```python
from build123d import *

# Parameters (mm, degrees)
F1_DEPTH = 3.5
F2_R     = 0.15
F4_DEPTH = 25


with BuildPart() as f1:
    # F0 (on Top) → F1 (new body)
    with BuildSketch(Plane.XY):
        with BuildLine():
            ThreePointArc((2.0309193372, 2.850502876), (0, 4.9428488608), (-2.0309193372, 2.850502876))
            ThreePointArc((-2.0309193372, 2.850502876), (0, -3.5), (2.0309193372, 2.850502876))
        make_face()
        with BuildLine():
            ThreePointArc((0.7830913136, 1.8403173625), (0, -2), (-0.7830913136, 1.8403173625))
            ThreePointArc((-0.7830913136, 1.8403173625), (0, 3.4622241035), (0.7830913136, 1.8403173625))
        make_face(mode=Mode.SUBTRACT)
    extrude(amount=F1_DEPTH)

    # F2
    f2_edges = [f1.edges().sort_by_distance(p)[0] for p in [
        (-0.783091, 1.840317, 1.75),
        (0.783091, 1.840317, 1.75),
    ]]
    fillet(f2_edges, radius=F2_R)

    # F3 (on Front) → F4 (cut)
    with BuildSketch(Plane.XZ):
        Polygon((-2.6012919649, 8.286720852), (-4.2398504038, 8.1655834162), (3.1280116344, -5.5110100095), (4.8318293002, -5.5110100095), align=None)
    extrude(amount=F4_DEPTH, mode=Mode.SUBTRACT)


solid = f1.part
```
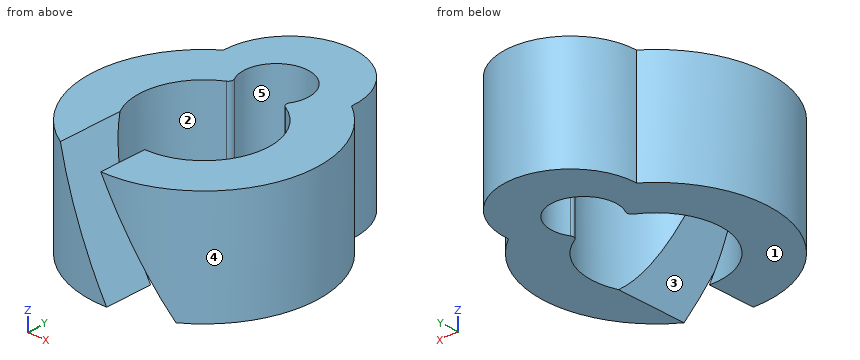
Input: part model. Units: mm. Frame: model coordinates. Face numbers are marked on the shaded views. A direction names the side the tool comes from. Give positions to 0.01 mm unless a question says otherwise; leave off trailing zeros. Write each loop counter-clockwise with the first axis right and the second up, starting at its lowest first coordinate (ties: lowest second). Pieces come first, ordered by that corner, then holes. Notation, with made-up numbers: (33.5, 17) - (57.5, 17) arc R15 ccw to (57.5, 26) - close; hole circle Ø1 at (72, -28). An arc over 180 degrees is marked (long way). Write item = value, one per line. Start each with the question number.
1. Ray query, L1, parallel to X at y = 0, z = 3; L2, parallel to Y at x = 0, z = 2.45; L3, parallel to X at y = -0.5, z = 1.85. Return the intervals inside material, ascending.
2. First-contact query: pin 1 Ø2 at (x, z) = (-1.5, 2) entering from +Y; pin 2 Ø2 at (y, z) = (3, 2.5) entering from +X. Flat tips, straight axial feed; report the tip coordinate or a pass-through.
3. Access query for the marked faces 1 and 2. Directions: +Z, -Z, +X, -X, +Y, -Y. A direction counts if a zero-diameter tool reaches every point of the face in a straight line with its end or side. Return the directions, or none.
4. Section query A-A, the plane y = 2.75. Output: boundary loops of the cut face in (x, z), then the cut area to 3 significant figures.
5. Section query C-C, the plane x = -3. Output: boundary loops of the cut face in (y, z).
6. Section query D-D, the plane x = 2.5. Output: boundary loops of the cut face in (y, z), then the cut area to 3 significant figures.
7. Section query B-B, the plane x = 1.75. Output: boundary loops of the cut face in (y, z).
8. Mould query, pull axis Y, two halves, no side actions, for the marked faces 3, 4 and 5. Classes: released by +Y, released by -Y, zero draft, split by the parting line, or undercut.
Check sheet entries:
q1.L1 = -3.5 to -2, 2 to 3.5
q1.L2 = 3.46 to 4.94
q1.L3 = -3.46 to -1.94, 1.94 to 3.46
q2.pin_1 = 4.88
q2.pin_2 = 2.87
q3.face_1 = -Z, +X, -X, +Y, -Y
q3.face_2 = +Z, -Z
q4.outline = (-2.17, 0) - (-0.96, 0) - (-0.96, 3.5) - (-2.17, 3.5) - close; (0.96, 0) - (2.17, 0) - (2.17, 3.5) - (0.96, 3.5) - close
q4.area = 8.45 mm2
q5.outline = (-1.8, 0) - (1.8, 0) - (1.8, 3.5) - (-1.8, 3.5) - close
q6.outline = (-2.45, 0) - (2.45, 0) - (2.45, 3.5) - (-2.45, 3.5) - close
q6.area = 17.1 mm2
q7.outline = (-3.03, 0.21) - (-0.97, 0.21) - (-0.97, 3.5) - (-3.03, 3.5) - close; (0.97, 0) - (3.94, 0) - (3.94, 3.5) - (0.97, 3.5) - close
q8.face_3 = zero draft
q8.face_4 = split by the parting line
q8.face_5 = undercut
